```python
from build123d import *

# Parameters (mm, degrees)
ESQUISSE1_W             = 200
ESQUISSE1_H             = 135
BOSS_EXTRU_1_DEPTH      = 727
COQUE1_T                = -10
ESQUISSE2_W             = 20
ESQUISSE2_H             = 500
ENL_V_MAT_EXTRU_1_DEPTH = 10
ESQUISSE3_W             = 200
ESQUISSE3_H             = 150
BOSS_EXTRU_2_DEPTH      = 20
CHANFREIN1_SIZE         = 15
ESQUISSE4_W             = 140
ESQUISSE4_H             = 75
ENL_V_MAT_EXTRU_2_DEPTH = 747.428328776
CONG_3_R                = 25
CONG_2_R                = 25
ENL_V_START             = -5
ENL_V_MAT_EXTRU_3_DEPTH = 5
ESQUISSE8_W             = 200
ESQUISSE8_H             = 135
BOSS_EXTRU_3_DEPTH      = 30
CONG_5_R                = 10


with BuildPart() as part:
    # Esquisse1 → Boss.-Extru.1 (new body)
    with BuildSketch(Plane.XY):
        Rectangle(ESQUISSE1_W, ESQUISSE1_H)
    extrude(amount=BOSS_EXTRU_1_DEPTH)

    # Coque1
    coque1_openings = [part.faces().sort_by_distance(p)[0] for p in [
        (0, 0, 0),
    ]]
    offset(amount=COQUE1_T, openings=coque1_openings, kind=Kind.INTERSECTION)

    # Esquisse2 → Enlèv. mat.-Extru.1 (cut)
    with BuildSketch(Plane.XZ.offset(67.5)):
        with Locations((-60, 457)):
            Rectangle(ESQUISSE2_W, ESQUISSE2_H)
        with Locations((60, 457)):
            Rectangle(ESQUISSE2_W, ESQUISSE2_H)
    extrude(amount=-ENL_V_MAT_EXTRU_1_DEPTH, mode=Mode.SUBTRACT)

    # Esquisse3 → Boss.-Extru.2 (add)
    with BuildSketch(Plane(origin=(0, 0, 0), x_dir=(-1, 0, 0), z_dir=(0, 0, -1))):
        with Locations((0, -142.5)):
            Rectangle(ESQUISSE3_W, ESQUISSE3_H)
    extrude(amount=-BOSS_EXTRU_2_DEPTH)

    # Chanfrein1
    chanfrein1_edges = [part.edges().sort_by_distance(p)[0] for p in [
        (0, -67.5, 20),
    ]]
    chamfer(chanfrein1_edges, length=CHANFREIN1_SIZE)

    # Esquisse4 → Enlèv. mat.-Extru.2 (cut, through all)
    with BuildSketch(Plane.XY.offset(20)):
        with Locations((0, -150)):
            Rectangle(ESQUISSE4_W, ESQUISSE4_H)
    extrude(amount=-ENL_V_MAT_EXTRU_2_DEPTH, mode=Mode.SUBTRACT)

    # Congé3
    cong_3_edges = [part.edges().sort_by_distance(p)[0] for p in [
        (70, -187.5, 10),
        (-70, -187.5, 10),
        (-70, -112.5, 10),
        (70, -112.5, 10),
    ]]
    fillet(cong_3_edges, radius=CONG_3_R)

    # Congé2
    cong_2_edges = [part.edges().sort_by_distance(p)[0] for p in [
        (-100, -217.5, 10),
        (100, -217.5, 10),
    ]]
    fillet(cong_2_edges, radius=CONG_2_R)

    # Esquisse5 → Enlèv. mat.-Extru.3 (cut)
    with BuildSketch(Plane.XY.offset(20).offset(ENL_V_START)):
        with BuildLine():
            Line((45, -102.5), (-45, -102.5))
            ThreePointArc((-45, -102.5), (-69.748737342, -112.751262658), (-80, -137.5))
            Line((-80, -137.5), (-80, -162.5))
            ThreePointArc((-80, -162.5), (-69.748737342, -187.248737342), (-45, -197.5))
            Line((-45, -197.5), (45, -197.5))
            ThreePointArc((45, -197.5), (69.748737342, -187.248737342), (80, -162.5))
            Line((80, -162.5), (80, -137.5))
            ThreePointArc((80, -137.5), (69.748737342, -112.751262658), (45, -102.5))
        make_face()
        with BuildLine():
            Line((70, -162.5), (70, -137.5))
            ThreePointArc((70, -137.5), (62.67766953, -119.82233047), (45, -112.5))
            Line((45, -112.5), (-45, -112.5))
            ThreePointArc((-45, -112.5), (-62.67766953, -119.82233047), (-70, -137.5))
            Line((-70, -137.5), (-70, -162.5))
            ThreePointArc((-70, -162.5), (-62.67766953, -180.17766953), (-45, -187.5))
            Line((-45, -187.5), (45, -187.5))
            ThreePointArc((45, -187.5), (62.67766953, -180.17766953), (70, -162.5))
        make_face(mode=Mode.SUBTRACT)
    extrude(amount=ENL_V_MAT_EXTRU_3_DEPTH, mode=Mode.SUBTRACT)

    # Esquisse8 → Boss.-Extru.3 (add)
    with BuildSketch(Plane.XY.offset(727)):
        Rectangle(ESQUISSE8_W, ESQUISSE8_H)
    extrude(amount=BOSS_EXTRU_3_DEPTH)

    # Congé5
    cong_5_edges = [part.edges().sort_by_distance(p)[0] for p in [
        (0, -67.5, 757),
        (100, -67.5, 396),
        (-100, -67.5, 396),
        (-100, 67.5, 378.5),
        (100, 67.5, 378.5),
    ]]
    fillet(cong_5_edges, radius=CONG_5_R)


solid = part.part
```
The model under review builds one solid part; all positions refer to its coordinate system, in mm. A direction names the side the tool comes from. Round coordinates to 2 decimals unless told otherwise and drop trailing zeros. Order: outer loops, then holes, each group sorted by start corner. A loop starts at its lowest first (then second) coordinate and runs counter-clockwise, first axis right, second up. Notation, with made-up numbers: (18, -17.75) - (50, -17.75) arc R26 ccw to (50, -3.75) - close; hole circle Ø7 at (-6, 69). An arc over 180 degrees is marked (long way). Answer in a Markdown table with one row per item.
(1) For line 1 (Y direction, x = -76, z = 139); line 2 (X direction, y = -42, z = 301); line 3 (X direction, y = -65, z = 456), list the stretches that pass through material, from the lowest coordinate up. Write a range as from..to.
Result set:
| item | result |
|---|---|
| line 1 | y = -67.5..-57.5, 57.5..67.5 |
| line 2 | x = -100..-90, 90..100 |
| line 3 | x = -96.61..-70, -50..50, 70..96.61 |
(2) Take a section at A-A on z = 332.5. Write out the cut boundary in (x, y).
Result set:
| item | result |
|---|---|
| outline | (-100, -57.5) arc R10 ccw to (-90, -67.5) - (-70, -67.5) - (-70, -57.5) - (-90, -57.5) - (-90, 57.5) - (90, 57.5) - (90, -57.5) - (70, -57.5) - (70, -67.5) - (90, -67.5) arc R10 ccw to (100, -57.5) - (100, 57.5) arc R10 ccw to (90, 67.5) - (-90, 67.5) arc R10 ccw to (-100, 57.5) - close; (-50, -67.5) - (50, -67.5) - (50, -57.5) - (-50, -57.5) - close |
(3) Machinability: for faces 4 (the face through (-1, -187.5, 8)), 5 (the face through (-90, -1, 353)), 6 (the face through (-1, -67.5, 386)), which of the approach directions +Z, -Z, +X, -X, +Y, -Y give a long, thin tool a straight path to every point of the face, cutting with its end or side? Answer none if there is none.
Result set:
| item | result |
|---|---|
| face 4 | +Z, -Z |
| face 5 | -Z |
| face 6 | +Z, +X, -X, -Y |
(4) Take a section at C-C on x = -13. Write out the cut boundary in (y, z).
Result set:
| item | result |
|---|---|
| outline | (-217.5, 0) - (-187.5, 0) - (-187.5, 15) - (-197.5, 15) - (-197.5, 20) - (-217.5, 20) - close; (-112.5, 0) - (-57.5, 0) - (-57.5, 717) - (57.5, 717) - (57.5, 0) - (67.5, 0) - (67.5, 757) - (-57.5, 757) arc R10 ccw to (-67.5, 747) - (-67.5, 35) - (-82.5, 20) - (-102.5, 20) - (-102.5, 15) - (-112.5, 15) - close |
(5) Mouldability with a two-part tool opening along X and no side actions: class faces 1 (the face through (-92.482, -210.371, 10.14)), 2 (the face through (-1, 67.5, 373)), 3 (the face through (-1, 1, 717)) as released by +X, released by -X, zero draft, split by the parting line, or undercut.
Result set:
| item | result |
|---|---|
| face 1 | released by -X |
| face 2 | zero draft |
| face 3 | undercut |
(6) Take a section at D-D on y = -150. Write out the cut boundary in (x, z).
Result set:
| item | result |
|---|---|
| outline | (-100, 0) - (-70, 0) - (-70, 15) - (-80, 15) - (-80, 20) - (-100, 20) - close; (70, 0) - (100, 0) - (100, 20) - (80, 20) - (80, 15) - (70, 15) - close |
(7) Clearance check with flat-ended pins moving along their axes: P1, Ø2, axis at x = -4, z = 245.5, coming from the -Y side; P2, Ø3, axis at y = -62, z = 533, coming from the +X side; P3, Ø3, axis at x = 56, y = -62.5, coming from the +Z side. State where each tip first meets the part, or that it passes through.
Result set:
| item | result |
|---|---|
| P1 | stops at y = -67.5 |
| P2 | stops at x = 99.54 |
| P3 | stops at z = 756.37 |
(8) Take a section at B-B on z = 176.5. Write out the cut boundary in (x, y), plus the area to 3 significant figures.
Result set:
| item | result |
|---|---|
| outline | (-100, -57.5) arc R10 ccw to (-90, -67.5) - (90, -67.5) arc R10 ccw to (100, -57.5) - (100, 57.5) arc R10 ccw to (90, 67.5) - (-90, 67.5) arc R10 ccw to (-100, 57.5) - close; hole (-90, -57.5) - (90, -57.5) - (90, 57.5) - (-90, 57.5) - close |
| area | 6,210 mm2 |
